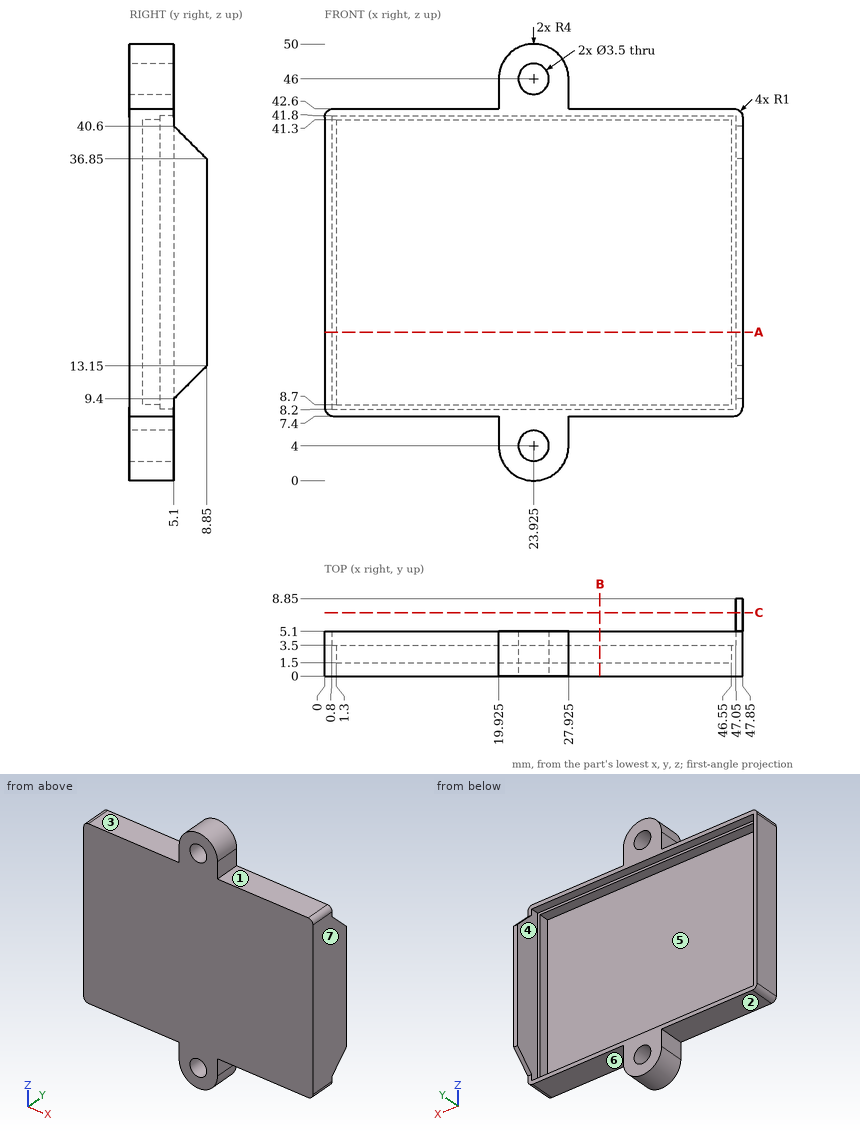
Could you check a few things on this drawing? It's one solid part, dimensions in mm from its lowest x, y, z. A direction names the side the tool comes from. Coordinates: 2 decimals unless noted, no trailing zeros. Loops run counter-clockwise (first coordinate to the right, second up) from the corner with the lowest first, then second, coordinate; pieces in that order, holes last. Notation, with made-up numbers: (25, -10) - (35, -10) arc R34 cw to (35, 26) - close; hole circle Ø5 at (-31, -6). An arc over 180 degrees is marked (long way). Answer as a JSON object with one key per item and string values. Group by question number.
Item 1: If we mould it in two halves opening along X, with no side actions, what happens to the marked faces 5, 6 and 7? For each: released by +X, released by -X, zero draft, split by the parting line, or undercut.
Item 2: If we section it at C-C (y = 7.25): List the corners of the cut face in (x, z) for me.
Item 3: If I drill on L1, parallel to X at y = 2.1, z = 4 (3 decimals); L2, parallel to Z at x = 24, y = 1; L3, parallel to Z at x = 18.5, y = 4, over which ranges is the centre line in solid material (lowest first)? Write a range as from..to.
Item 4: If we section it at A-A (z = 17): List the corners of the cut face in (x, y) for me.
Item 5: On a 3-axis mill with a long thin cutter (end or side, diameter ignored), from which of +Z, -Z, +X, -X, +Y, -Y can I reach the whole of each face in a straight line? I mean the marked faces 1, 2, 3 and 4. Say none if no direction works.
Item 6: If we section it at B-B (x = 31.5): List the corners of the cut face in (y, z) for me.
Item 7: For pin 1 (1.5 mm diameter, centred on x = 14, y = 2, fed in from -Z); pin 2 (2 mm diameter, centred on x = 28, y = 2, fed in from -Z); pin 3 (1.6 mm diameter, centred on y = 3, z = 31.5, fed in from -X); pin 4 (1 mm diameter, centred on y = 3.5, z = 5.5, fed in from -X) (3 decimals), each with a flat end and sliding along its axis, tell me the tip position at first contact or that it passes through.
Returned:
{
 "1": {"face 5": "undercut", "face 6": "zero draft", "face 7": "released by +X"},
 "2": {"outline": "(47.05, 11.55) - (47.85, 11.55) - (47.85, 38.45) - (47.05, 38.45) - close"},
 "3": {"L1": "x = 19.925..22.175, 25.675..27.925", "L2": "z = 0..2.25, 5.75..44.25, 47.75..50", "L3": "z = 7.4..8.2, 41.8..42.6"},
 "4": {"outline": "(0, 0) - (47.85, 0) - (47.85, 8.85) - (47.05, 8.85) - (47.05, 3.5) - (46.55, 3.5) - (46.55, 1.5) - (1.3, 1.5) - (1.3, 3.5) - (0.8, 3.5) - (0.8, 5.1) - (0, 5.1) - close"},
 "5": {"face 1": "+Z, +X, +Y, -Y", "face 2": "-Z, -X, +Y, -Y", "face 3": "+Z, -X, +Y, -Y", "face 4": "+Y"},
 "6": {"outline": "(0, 7.4) - (5.1, 7.4) - (5.1, 8.2) - (3.5, 8.2) - (3.5, 8.7) - (1.5, 8.7) - (1.5, 41.3) - (3.5, 41.3) - (3.5, 41.8) - (5.1, 41.8) - (5.1, 42.6) - (0, 42.6) - close"},
 "7": {"pin 1": "stops at z = 7.4", "pin 2": "stops at z = 1.44", "pin 3": "stops at x = 0", "pin 4": "stops at x = 19.925"}
}
